Here's how the part is built. I have some questions about the finished solid (model axes, mm). Face numbers are marked on the shaded views. Give positions to 0.01 mm unless a question says otherwise; leave off trailing zeros. Loops run counter-clockwise (first coordinate to the right, second up) from the corner with the lowest first, then second, coordinate; pieces in that order, holes last.
Q1. I need wall thicknesses on probe 1 along X at (y, z) = (52, 5.75); probe 2 along Y at (x, z) = (80, 4.75); probe 3 along Y at (x, z) = (18, 4.5). Which ranges of each line are inside material? Lowest first, please.
Q2. Suppose I cut it at D-D (x = 81). List the corners of the cut face in (y, z) for me.
Q3. I'm going to push a flat-ended pin straight in: P1, Ø17.5, axis at x = 50, y = 51, coming from the +Z side. Where does the tip first touch, or does it pass through?
Q4. Suppose I cut it at A-A (x = 20). List the corners of the cut face in (y, z) for me.
Q5. Suppose I cut it at C-C (z = 3). List the corners of the cut face in (x, y) for me.
Q6. Thinking about a two-plate mould opening in Y: for the marked faces 1, 2 and 3, which applies, pulls with the +Y half, pulls with the -Y half, needs draft (parallel to the pull), parting line crosses it, or undercut?
Q7. Suppose I cut it at B-B (y = 54). List the corners of the cut face in (x, z) for me.
Autodesk Inventor part; units mm, degrees
ref_plane "YZ Plane" through (0, 0, 0) normal (1, 0, 0) x (0, 1, 0)
ref_plane "XZ Plane" through (0, 0, 0) normal (0, 1, 0) x (-1, 0, 0)
ref_plane "XY Plane" through (0, 0, 0) normal (0, 0, 1) x (1, 0, 0)
sketch "Boceto1" plane through (0, 0, 0) normal (0, 0, 1) x (1, 0, 0)
  line L0 (0, 0) -> (100, 0)
  line L1 (100, 0) -> (100, 61)
  line L2 (100, 61) -> (0, 61)
  line L3 (0, 61) -> (0, 0)
  dimension "d0" = 61
  dimension "d1" = 100
extrude "Extrusión1" add sketch "Boceto1" along normal blind 18
sketch "Boceto2" plane through (0, 0, 18) normal (0, 0, 1) x (1, 0, 0)
  circle A0 centre (50, 51) radius 11
  line L0 (0, 61) -> (0, 0)
  line L1 (100, 61) -> (0, 61)
  line L2 (50, 51) -> (20, 51) construction
  circle A1 centre (20, 51) radius 4
  line L3 (50, 51) -> (50, 22.8333) construction
  circle A2 centre (80, 51) radius 4
  circle A3 centre (29.5218, 59.04) radius 1.5
  circle A4 centre (50, 51) radius 22 construction
  line L4 (29.5218, 59.04) -> (50, 51) construction
  line L5 (50, 51) -> (78.6691, 39.7442) construction
  circle A5 centre (70.4782, 42.96) radius 1.5
  line L6 (50, 51) -> (39.4009, 24.0037) construction
  circle A6 centre (41.96, 30.5218) radius 1.5
  point P0 (54.5826, 61)
  point P1 (45.4174, 61)
  dimension "d4" = 22
  dimension "d5" = 50
  dimension "d6" = 10
  dimension "d7" = 8
  dimension "d8" = 30
  dimension "d9" = 3
  dimension "d10" = 1.96
  dimension "d11" = 44
  dimension "d12" = 3
  dimension "d13" = 90
  dimension "d14" = 3
extrude "Extrusión2" cut sketch "Boceto2" against normal blind 18 contours A0 L1 | A1 | A2 | A3 | A6 picked at (46.6624, 53.5107)
sketch "Boceto3" plane through (0, 0, 18) normal (0, 0, 1) x (1, 0, 0)
  point P0 (0, 0)
sketch "Boceto4" plane through (0, 0, 0) normal (0, 0, -1) x (-1, 0, 0)
  arc A0 (-54.5826, 61) -> (-45.4174, 61) centre (-50, 51) ccw
  arc A1 (-54.5826, 61) -> (-45.4174, 61) centre (-50, 51) ccw
  circle A2 centre (-41.96, 30.5218) radius 1.5
  circle A3 centre (-41.96, 30.5218) radius 1.5
  circle A4 centre (-29.5218, 59.04) radius 1.5
  circle A5 centre (-29.5218, 59.04) radius 1.5
  line L0 (-45.4174, 61) -> (0, 61)
  line L1 (-45.4174, 61) -> (-54.5826, 61)
  point P0 (0, 0)
extrude "Extrusión3" add sketch "Boceto4" against normal blind 7 contours L1 A0
sketch "Boceto5" plane through (0, 0, 18) normal (0, 0, 1) x (1, 0, 0)
  circle A0 centre (29.5218, 59.04) radius 1.5
  circle A1 centre (29.5218, 59.04) radius 1.5
  circle A2 centre (41.96, 30.5218) radius 1.5
  circle A3 centre (41.96, 30.5218) radius 1.5
  point P0 (0, 0)
extrude "Extrusión4" add sketch "Boceto5" against normal up to surface (18 mm away)
properties part number "013" material "CFRP"
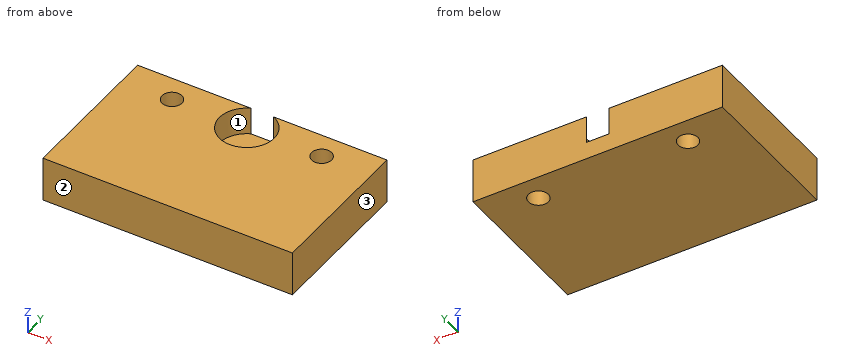
Solutions:
1. probe 1: x = 0 to 16.13, 23.87 to 76.13, 83.87 to 100
1. probe 2: y = 0 to 47, 55 to 61
1. probe 3: y = 0 to 47.54, 54.46 to 61
2. outline: (0, 0) - (47.13, 0) - (47.13, 18) - (0, 18) - close; (54.87, 0) - (61, 0) - (61, 18) - (54.87, 18) - close
3. P1: stops at z = 7
4. outline: (0, 0) - (47, 0) - (47, 18) - (0, 18) - close; (55, 0) - (61, 0) - (61, 18) - (55, 18) - close
5. outline: (0, 0) - (100, 0) - (100, 61) - (0, 61) - close; hole circle Ø8 at (20, 51); hole circle Ø8 at (80, 51)
6. face 1: undercut
6. face 2: pulls with the -Y half
6. face 3: needs draft
7. outline: (0, 0) - (17.35, 0) - (17.35, 18) - (0, 18) - close; (22.65, 0) - (77.35, 0) - (77.35, 18) - (60.58, 18) - (60.58, 7) - (39.42, 7) - (39.42, 18) - (22.65, 18) - close; (82.65, 0) - (100, 0) - (100, 18) - (82.65, 18) - close
